Verification items for the finished model (mm, model axes). A direction names the side the tool comes from. Coordinates: 2 decimals unless noted, no trailing zeros. Order: outer loops, then holes, each group sorted by start corner. A loop starts at its lowest first (then second) coordinate and runs counter-clockwise, first axis right, second up. Notation, with made-up numbers: M 43,-14 L 53,-14 A15 cw 53,-7 Z; hole C 52.25,85.5 d3. An arc over 180 degrees is marked long. Answer as a JSON object with one key per item and string values. Group by question number.
(1) Access from +Z, -Z, +X, -X, +Y, -Y to the whole of each face (thin tool, end or side, straight path). Record for faces 5 (the face through (-2, 0, -2)), 6 (the face through (61.379, 3.219, -114.297)).
(2) Cross-section at B-B (x = -61.1). Enter the section's corners in (y, z), plus the area to 3 significant figures.
(3) Cross-section at C-C (y = 5). Count the separate pieces of the cut face and the enclosed holes in it, plus the area to 3 significant figures.
(4) Cross-section at A-A (z = -18.5). Enter the section's corners in (x, y).
(5) Material ranges on line 1 (X direction, y = 5.75, z = 20.5); line 2 (Z direction, x = 0.5, y = 0.75); line 3 (X direction, y = 4.75, z = 99.5), recorded low to high.
(6) Mould release check, pull along X, two halves, no side actions. Record for faces 1 (the face through (60.821, 3.219, 114.297)), 2 (the face through (142.36, 3.22, 142.76)), 3 (the face through (-142.76, 3.22, -142.36)), 4 (the face through (-2, 6.35, -2)): released by +X, released by -X, zero draft, split by the parting line, or undercut.
from build123d import *

# Parameters (mm, degrees)
SKETCH1_W           = 300
SKETCH1_H           = 300
BOSS_EXTRUDE1_DEPTH = 6.35
SKETCH2_R           = 2.0828
SKETCH2_W           = 25.4
SKETCH2_H           = 63.5
CUT_EXTRUDE1_DEPTH  = 213.227054119
FILLET1_R           = 25.4


with BuildPart() as part:
    # Sketch1 → Boss-Extrude1 (new body)
    with BuildSketch(Plane(origin=(0, 0, 0), x_dir=(1, 0, 0), z_dir=(0, 1, 0))):
        Rectangle(SKETCH1_W, SKETCH1_H)
    extrude(amount=BOSS_EXTRUDE1_DEPTH)

    # Sketch2 → Cut-Extrude1 (cut, through all)
    with BuildSketch(Plane(origin=(0, 6.35, 0), x_dir=(1, 0, 0), z_dir=(0, 1, 0))):
        with Locations(Location((-87.138207153, 87.138207153, 0), (0, 0, 270))):
            Circle(SKETCH2_R)
        with Locations(Location((87.138207153, 87.138207153, 0), (0, 0, 90))):
            Circle(SKETCH2_R)
        with Locations(Location((87.138207153, -87.138207153, 0), (0, 0, 270))):
            Circle(SKETCH2_R)
        with Locations(Location((-87.138207153, -87.138207153, 0), (0, 0, 90))):
            Circle(SKETCH2_R)
        with Locations(Location((-141.6688, 99.2, 0), (0, 0, 270))):
            Circle(SKETCH2_R)
        with Locations(Location((-141.6688, 61.1, 0), (0, 0, 270))):
            Circle(SKETCH2_R)
        with Locations(Location((-141.6688, -99.2, 0), (0, 0, 270))):
            Circle(SKETCH2_R)
        with Locations(Location((-141.6688, -61.1, 0), (0, 0, 270))):
            Circle(SKETCH2_R)
        with Locations(Location((-76.2, -141.6688, 0), (0, 0, 270))):
            Circle(SKETCH2_R)
        with Locations(Location((76.2, -141.6688, 0), (0, 0, 270))):
            Circle(SKETCH2_R)
        with Locations(Location((0, -141.6688, 0), (0, 0, 270))):
            Circle(SKETCH2_R)
        with Locations(Location((-76.2, 141.6688, 0), (0, 0, 270))):
            Circle(SKETCH2_R)
        with Locations(Location((0, 141.6688, 0), (0, 0, 270))):
            Circle(SKETCH2_R)
        with Locations(Location((76.2, 141.6688, 0), (0, 0, 270))):
            Circle(SKETCH2_R)
        with Locations(Location((141.6688, 99.2, 0), (0, 0, 270))):
            Circle(SKETCH2_R)
        with Locations(Location((141.6688, 61.1, 0), (0, 0, 270))):
            Circle(SKETCH2_R)
        with Locations(Location((141.6688, -99.2, 0), (0, 0, 270))):
            Circle(SKETCH2_R)
        with Locations(Location((141.6688, -61.1, 0), (0, 0, 270))):
            Circle(SKETCH2_R)
        with Locations(Location((-139.6622, 40.4492, 0), (0, 0, 270))):
            Circle(SKETCH2_R)
        with Locations(Location((-124.7778, 40.4492, 0), (0, 0, 270))):
            Circle(SKETCH2_R)
        with Locations(Location((-139.6622, -40.2212, 0), (0, 0, 270))):
            Circle(SKETCH2_R)
        with Locations(Location((-124.7778, -40.2212, 0), (0, 0, 270))):
            Circle(SKETCH2_R)
        with Locations(Location((124.7778, 40.4492, 0), (0, 0, 270))):
            Circle(SKETCH2_R)
        with Locations(Location((139.6622, 40.4492, 0), (0, 0, 270))):
            Circle(SKETCH2_R)
        with Locations(Location((124.7778, -40.2212, 0), (0, 0, 270))):
            Circle(SKETCH2_R)
        with Locations(Location((139.6622, -40.2212, 0), (0, 0, 270))):
            Circle(SKETCH2_R)
        with BuildLine():
            Line((-73.8, -101.6), (-73.8, 101.6))
            ThreePointArc((-73.8, 101.6), (-61.1, 114.3), (-48.4, 101.6))
            Line((-48.4, 101.6), (-48.4, -101.6))
            ThreePointArc((-48.4, -101.6), (-61.1, -114.3), (-73.8, -101.6))
        make_face()
        with BuildLine():
            Line((73.8, -101.6), (73.8, 101.6))
            ThreePointArc((73.8, 101.6), (61.1, 114.3), (48.4, 101.6))
            Line((48.4, 101.6), (48.4, -101.6))
            ThreePointArc((48.4, -101.6), (61.1, -114.3), (73.8, -101.6))
        make_face()
        with Locations((132.219999974, 0)):
            Rectangle(SKETCH2_W, SKETCH2_H)
        with Locations((-132.219999974, 0)):
            Rectangle(SKETCH2_W, SKETCH2_H)
    extrude(amount=-CUT_EXTRUDE1_DEPTH, mode=Mode.SUBTRACT)

    # Fillet1
    fillet1_edges = [part.edges().sort_by_distance(p)[0] for p in [
        (150, 3.175, 150),
        (-150, 3.175, 150),
        (-150, 3.175, -150),
        (150, 3.175, -150),
    ]]
    fillet(fillet1_edges, radius=FILLET1_R)


solid = part.part
Taken from the geometry:
{
 "1": {"face 5": "+Z, -Z, +X, -X, -Y", "face 6": "+Y, -Y"},
 "2": {"outline": "M 0,-150 L 6.35,-150 L 6.35,-114.3 L 0,-114.3 Z; M 0,114.3 L 6.35,114.3 L 6.35,150 L 0,150 Z", "area": "453 mm²"},
 "3": {"separate pieces": "1", "enclosed holes": "30", "area": "74,500 mm²"},
 "4": {"outline": "M -150,0 L -144.92,0 L -144.92,6.35 L -150,6.35 Z; M -119.52,0 L -73.8,0 L -73.8,6.35 L -119.52,6.35 Z; M -48.4,0 L 48.4,0 L 48.4,6.35 L -48.4,6.35 Z; M 73.8,0 L 119.52,0 L 119.52,6.35 L 73.8,6.35 Z; M 144.92,0 L 150,0 L 150,6.35 L 144.92,6.35 Z"},
 "5": {"line 1": "x = -150 to -144.92, -119.52 to -73.8, -48.4 to 48.4, 73.8 to 119.52, 144.92 to 150", "line 2": "z = -150 to -143.69, -139.65 to 139.65, 143.69 to 150", "line 3": "x = -150 to -143.73, -139.61 to -73.8, -48.4 to 48.4, 73.8 to 139.61, 143.73 to 150"},
 "6": {"face 1": "undercut", "face 2": "released by +X", "face 3": "released by -X", "face 4": "zero draft"}
}
